Autodesk Inventor part; units mm, degrees
ref_plane "YZ Plane" through (0, 0, 0) normal (1, 0, 0) x (0, 1, 0)
ref_plane "XZ Plane" through (0, 0, 0) normal (0, 1, 0) x (-1, 0, 0)
ref_plane "XY Plane" through (0, 0, 0) normal (0, 0, 1) x (1, 0, 0)
sketch "スケッチ1" plane through (0, 0, 0) normal (0, 0, 1) x (1, 0, 0)
  line L0 (0, 2.8868) -> (2.5, 1.4434)
  line L1 (2.5, 1.4434) -> (2.5, -1.4434)
  line L2 (2.5, -1.4434) -> (0, -2.8868)
  line L3 (0, -2.8868) -> (-2.5, -1.4434)
  line L4 (-2.5, -1.4434) -> (-2.5, 1.4434)
  line L5 (-2.5, 1.4434) -> (0, 2.8868)
  point P0 (0, 0)
  point P1 (0, 0)
  dimension "d0" = 5
extrude "押し出し1" add sketch "スケッチ1" along normal blind 16
sketch "スケッチ2" plane through (0, 0, 16) normal (0, 0, 1) x (1, 0, 0)
  circle A0 centre (0, 0) radius 1.3
  dimension "d3" = 2.6
extrude "押し出し2" add sketch "スケッチ2" along normal blind 5
thread "ねじ1"
sketch "スケッチ3" plane through (0, 0, 0) normal (0, 0, -1) x (-1, 0, 0)
  point P0 (0, 0)
hole "穴1" at (0, 0, 0) direction (0, 0, 1) diameter 2.113 depth 6 tip angle 118
properties part number "ジュラコンスペーサー（六角）_BS-2616E" material "アセタール樹脂、白"
Input: part model. Units: mm. Frame: model coordinates. A direction names the side the tool comes from. Round coordinates to 2 decimals unless told otherwise and drop trailing zeros. Loops run counter-clockwise (first coordinate to the right, second up) from the corner with the lowest first, then second, coordinate; pieces in that order, holes last. Notation, with made-up numbers: (-7, 20) -> (45, 20) arc R26 ccw to (45, 48) -> close; hole circle Ø9 at (29.25, -9). An arc over 180 degrees is marked (long way). Use one line per item in the form item = value. Start each with the question number.
Item 1: Mould query, pull axis X, two halves, no side actions, for faces 1 (the face through (-0.17, -1.29, 18.46)), 2 (the face through (-2.5, 0, 8)), 3 (the face through (-0.112, -0.146, 6.525)). Classes: pulls with the +X half, pulls with the -X half, needs draft (parallel to the pull), parting line crosses it, or undercut.
Item 2: Section query B-B on z = 15.5. Return the cut outline in (x, y).
Item 3: Material intervals for L1, parallel to X at y = 0, z = 2.2; L2, parallel to Z at x = -0.2, y = 2; L3, parallel to Y at x = -1.85, z = 1.5, sorted ascending. Write a range as from..to.
Item 4: Set-up query: faces 4 (the face through (1.03, -0.23, 3.04)), 5 (the face through (0, 0, 21)). Return all of +Z, -Z, +X, -X, +Y, -Y with unobstructed straight access to the full face (end or side cutting, diameter ignored); none if empty.
Item 5: Section query C-C on y = 1.7. Return the cut outline in (x, z), then the cut area to 3 significant figures.
Item 6: Section query D-D on x = -2. Return the cut outline in (y, z).
Item 7: Section query A-A on z = 1.5. Return the cut outline in (x, y), then the cut area to 3 significant figures.
Item 8: Contact query for a flat-ended pin moving along its axis: pin 1 Ø1.7 at (x, y) = (0, 0) entering from -Z. Output: stop coordinate, or through.
Ans:
q1.face_1 = parting line crosses it
q1.face_2 = pulls with the -X half
q1.face_3 = undercut
q2.outline = (-2.5, -1.44) -> (0, -2.89) -> (2.5, -1.44) -> (2.5, 1.44) -> (0, 2.89) -> (-2.5, 1.44) -> close
q3.L1 = -2.5..-1.06, 1.06..2.5
q3.L2 = 0..16
q3.L3 = -1.82..1.82
q4.face_4 = -Z
q4.face_5 = +Z, +X, -X, +Y, -Y
q5.outline = (-2.06, 0) -> (2.06, 0) -> (2.06, 16) -> (-2.06, 16) -> close
q5.area = 65.8 mm^2
q6.outline = (-1.73, 0) -> (1.73, 0) -> (1.73, 16) -> (-1.73, 16) -> close
q7.outline = (-2.5, -1.44) -> (0, -2.89) -> (2.5, -1.44) -> (2.5, 1.44) -> (0, 2.89) -> (-2.5, 1.44) -> close; hole circle Ø2.11 at (0, 0)
q7.area = 18.1 mm^2
q8.pin_1 = 6.12
